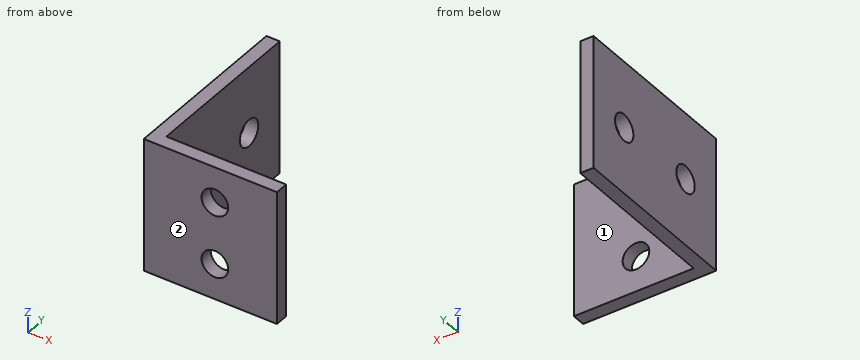
```python
from build123d import *

# Parameters (mm, degrees)
EXTRUSION1_DEPTH = 15
ESQUISSE2_R      = 1.5
EXTRUSION2_DEPTH = 15
ESQUISSE3_R      = 1.5
EXTRUSION3_DEPTH = 15


with BuildPart() as part:
    # Esquisse1 → Extrusion1 (new body)
    with BuildSketch(Plane.XY):
        Polygon((-28.567581117, 0.000842105), (-28.567581117, -19.999157895), (-13.567581117, -19.999157895), (-13.567581117, -18.499157895), (-27.067581117, -18.499157895), (-27.067581117, 0.000842105), align=None)
    extrude(amount=EXTRUSION1_DEPTH)

    # Esquisse2 → Extrusion2 (cut)
    with BuildSketch(Plane(origin=(0, -18.499157895, 0), x_dir=(-1, 0, 0), z_dir=(0, 1, 0))):
        with Locations((20.567581117, 4)):
            Circle(ESQUISSE2_R)
        with Locations((20.567581117, 11)):
            Circle(ESQUISSE2_R)
    extrude(amount=-EXTRUSION2_DEPTH, mode=Mode.SUBTRACT)

    # Esquisse3 → Extrusion3 (cut)
    with BuildSketch(Plane(origin=(-27.067581117, 0, 0), x_dir=(0, 0, -1), z_dir=(1, 0, 0))):
        with Locations(Location((-7.5, -4.999157895, 0), (0, 0, 90))):
            Circle(ESQUISSE3_R)
        with Locations(Location((-7.5, -14.999157895, 0), (0, 0, 90))):
            Circle(ESQUISSE3_R)
    extrude(amount=-EXTRUSION3_DEPTH, mode=Mode.SUBTRACT)


solid = part.part
```
Geometry check sheet. Reference: the model listing, model coordinates, mm. Face numbers are marked on the shaded views. A direction names the side the tool comes from. Coordinates: 2 decimals unless noted, no trailing zeros. Write each loop counter-clockwise with the first axis right and the second up, starting at its lowest first coordinate (ties: lowest second). Pieces come first, ordered by that corner, then holes. Notation, with made-up numbers: M -24.5,-35.5 L -3.5,-35.5 A36 cw -3.5,1.5 Z; hole C -10.75,-35.5 d8. An arc over 180 degrees is marked long. Answer as a JSON object with one key per item and string values.
1. Section check B-B, the plane y = -6. Enter the section's corners in (x, z).
Answers below:
{"outline": "M -28.57,0 L -27.07,0 L -27.07,6.38 L -28.57,6.38 Z; M -28.57,8.62 L -27.07,8.62 L -27.07,15 L -28.57,15 Z"}
2. Tool access check on the marked faces 1 and 2. Record the directions out of +Z, -Z, +X, -X, +Y, -Y that give a thin tool (end or side, any length) a straight path to the whole face; none if there is none.
Answers below:
{"face 1": "+Z, -Z, +X, +Y", "face 2": "+Z, -Z, +X, -X, -Y"}
3. Section check D-D, the plane x = -20.25. Enter the section's corners in (y, z).
Answers below:
{"outline": "M -20,0 L -18.5,0 L -18.5,2.53 L -20,2.53 Z; M -20,5.47 L -18.5,5.47 L -18.5,9.53 L -20,9.53 Z; M -20,12.47 L -18.5,12.47 L -18.5,15 L -20,15 Z"}
4. Scan lines: L1, parallel to Y at x = -27.25, z = 7.25; L2, parallel to Z at x = -21, y = -19; L3, parallel to X at y = -17.25, z = 3.25. Record each from-to range of solid material in increasing order.
Answers below:
{"L1": "y = -20 to -16.48, -13.52 to -6.48, -3.52 to 0", "L2": "z = 0 to 2.56, 5.44 to 9.56, 12.44 to 15", "L3": "x = -28.57 to -27.07"}
5. Go/stop test with flat-tipped pins: pin 1 Ø7.5 at (y, z) = (-9.5, 10) entering from +X; pin 2 Ø4 at (x, z) = (-20.57, 11) entering from +Y; pin 3 Ø2.5 at (y, z) = (-5, 7.5) entering from -X; pin 4 Ø3.5 at (x, z) = (-20.57, 4) entering from -Y. Record where each tip stops, or that it passes through.
Answers below:
{"pin 1": "stops at x = -27.07", "pin 2": "stops at y = -18.5", "pin 3": "passes through", "pin 4": "stops at y = -20"}
6. Section check A-A, the plane z = 7.5. Enter the section's corners in (x, y), plus the area to 4 significant figures.
Answers below:
{"outline": "M -28.57,-20 L -13.57,-20 L -13.57,-18.5 L -27.07,-18.5 L -27.07,-16.5 L -28.57,-16.5 Z; M -28.57,-13.5 L -27.07,-13.5 L -27.07,-6.5 L -28.57,-6.5 Z; M -28.57,-3.5 L -27.07,-3.5 L -27.07,0 L -28.57,0 Z", "area": "41.25 mm²"}
7. Section check C-C, the plane z = 11. Enter the section's corners in (x, y).
Answers below:
{"outline": "M -28.57,-20 L -22.07,-20 L -22.07,-18.5 L -27.07,-18.5 L -27.07,0 L -28.57,0 Z; M -19.07,-20 L -13.57,-20 L -13.57,-18.5 L -19.07,-18.5 Z"}
